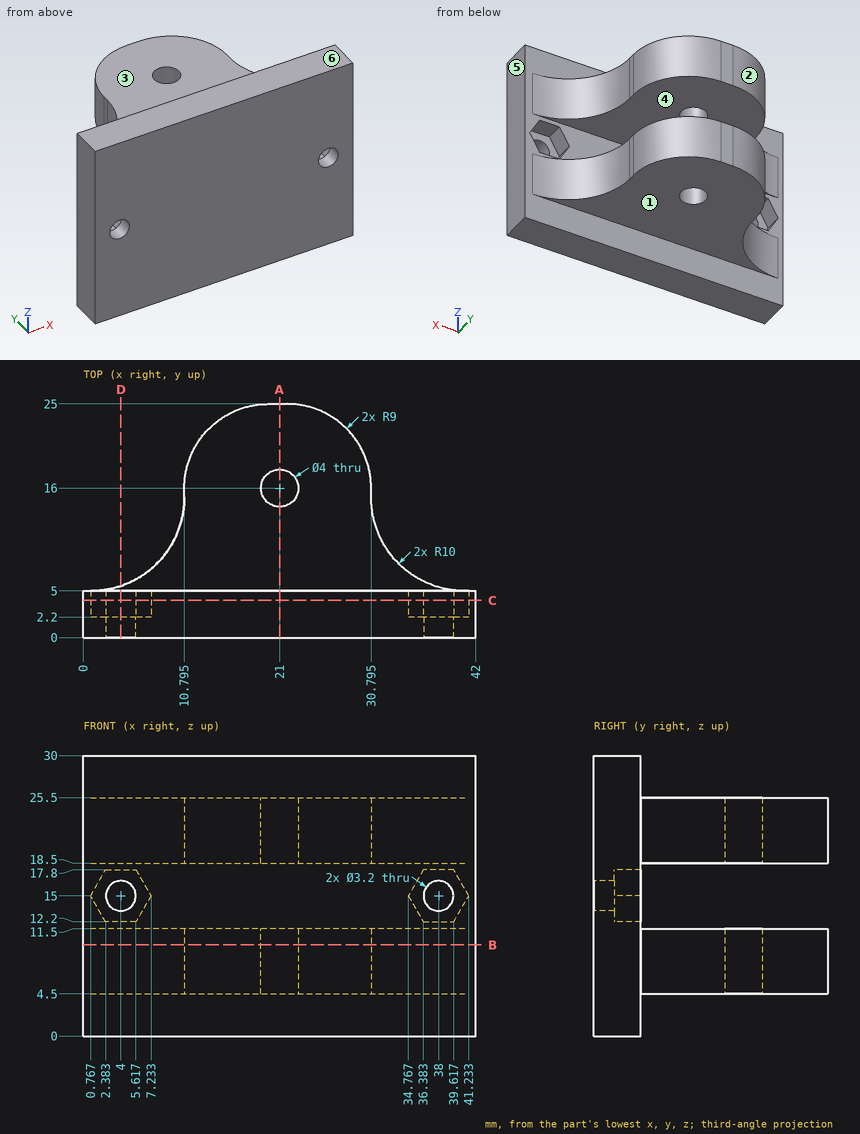
Design review of the part shown in the three views and the two pictorial views. Dimensions are in mm from the part's minimum x, y and z. A direction names the side the tool comes from. Give positions to 0.01 mm unless a question says otherwise; leave off trailing zeros. Write each loop counter-clockwise with the first axis right and the second up, starting at its lowest first coordinate (ties: lowest second). Pieces come first, ordered by that corner, then holes. Notation, with made-up numbers: (27.25, 16.25) -> (56.25, 16.25) arc R17 cw to (56.25, 26.25) -> close; hole circle Ø10 at (28, 43). An arc over 180 degrees is marked (long way). Answer in a Markdown table with one row per item.
1) Add section B-B on z = 9.75. State the section outline as (x, y) points (1 decimal).
Worked answers:
| item | result |
|---|---|
| outline | (0, 0) -> (42, 0) -> (42, 5) -> (40.8, 5) arc R10 cw to (30.8, 15) -> (30.8, 16) arc R9 ccw to (21.8, 25) -> (19.8, 25) arc R9 ccw to (10.8, 16) -> (10.8, 15) arc R10 cw to (0.8, 5) -> (0, 5) -> close; hole circle Ø4 at (21, 16) |
2) Tool access review of the marked faces 1, 2 and 3: name each direction out of +Z, -Z, +X, -X, +Y, -Y from which nothing blocks a thin tool from reaching the whole face with its end or side.
Worked answers:
| item | result |
|---|---|
| face 1 | -Z, +X, -X, +Y |
| face 2 | +Z, -Z, -X, +Y |
| face 3 | +Z, +X, -X, +Y |
3) Clearance check with flat-ended pins moving along their axes: P1, Ø0.8, axis at y = 15.5, z = 7, coming from the -X side (1 decimal); P2, Ø4, axis at x = 29.5, y = 20.5, coming from the +Z side; P3, Ø10, axis at x = 21.5, y = 14, coming from the -Z side. State where each tip first meets the part, or that it passes through.
Worked answers:
| item | result |
|---|---|
| P1 | x = 10.8 |
| P2 | z = 25.5 |
| P3 | z = 4.5 |
4) Mouldability with a two-part tool opening along Z and no side actions: class the marked faces 4, 5 and 6 as +Z half, -Z half, draft (parallel to the pull), parting line (faces both ways), or undercut.
Worked answers:
| item | result |
|---|---|
| face 4 | undercut |
| face 5 | draft |
| face 6 | +Z half |
5) Add section C-C on y = 4. State the section outline as (x, z) points.
Worked answers:
| item | result |
|---|---|
| outline | (0, 0) -> (42, 0) -> (42, 30) -> (0, 30) -> close; hole (0.77, 15) -> (2.38, 12.2) -> (5.62, 12.2) -> (7.23, 15) -> (5.62, 17.8) -> (2.38, 17.8) -> close; hole (34.77, 15) -> (36.38, 12.2) -> (39.62, 12.2) -> (41.23, 15) -> (39.62, 17.8) -> (36.38, 17.8) -> close |
6) For L1, parallel to Z at x = 38, y = 3.75; L2, parallel to Y at x = 21, z = 23.75; L3, parallel to Z at x = 30, y = 17.5, list the stretches that pass through material, from the lowest coordinate up. Write a range as [from, to].
Worked answers:
| item | result |
|---|---|
| L1 | [0, 12.2], [17.8, 30] |
| L2 | [0, 14], [18, 25] |
| L3 | [4.5, 11.5], [18.5, 25.5] |
7) Add section A-A on x = 21. State the section outline as (y, z) points, plus the area to 3 significant figures.
Worked answers:
| item | result |
|---|---|
| outline | (0, 0) -> (5, 0) -> (5, 4.5) -> (14, 4.5) -> (14, 11.5) -> (5, 11.5) -> (5, 18.5) -> (14, 18.5) -> (14, 25.5) -> (5, 25.5) -> (5, 30) -> (0, 30) -> close; (18, 4.5) -> (25, 4.5) -> (25, 11.5) -> (18, 11.5) -> close; (18, 18.5) -> (25, 18.5) -> (25, 25.5) -> (18, 25.5) -> close |
| area | 374 mm² |
8) Add section D-D on x = 4. State the section outline as (y, z) points.
Worked answers:
| item | result |
|---|---|
| outline | (0, 0) -> (5, 0) -> (5, 4.5) -> (5.53, 4.5) -> (5.53, 11.5) -> (5, 11.5) -> (5, 12.2) -> (2.2, 12.2) -> (2.2, 13.4) -> (0, 13.4) -> close; (0, 16.6) -> (2.2, 16.6) -> (2.2, 17.8) -> (5, 17.8) -> (5, 18.5) -> (5.53, 18.5) -> (5.53, 25.5) -> (5, 25.5) -> (5, 30) -> (0, 30) -> close |
